For this review, use the dimensioned drawing (mm, ordinates from the lowest corner) and the shaded views. A direction names the side the tool comes from. Coordinates: 2 decimals unless noted, no trailing zeros. Order: outer loops, then holes, each group sorted by start corner. A loop starts at its lowest first (then second) coordinate and runs counter-clockwise, first axis right, second up. Notation, with made-up numbers: M 41.25,22.25 L 83.25,22.25 A3 ccw 83.25,27.25 Z; hole C 65,11 d1. An arc over 180 degrees is marked long. Answer in a Markdown table with one row per item.
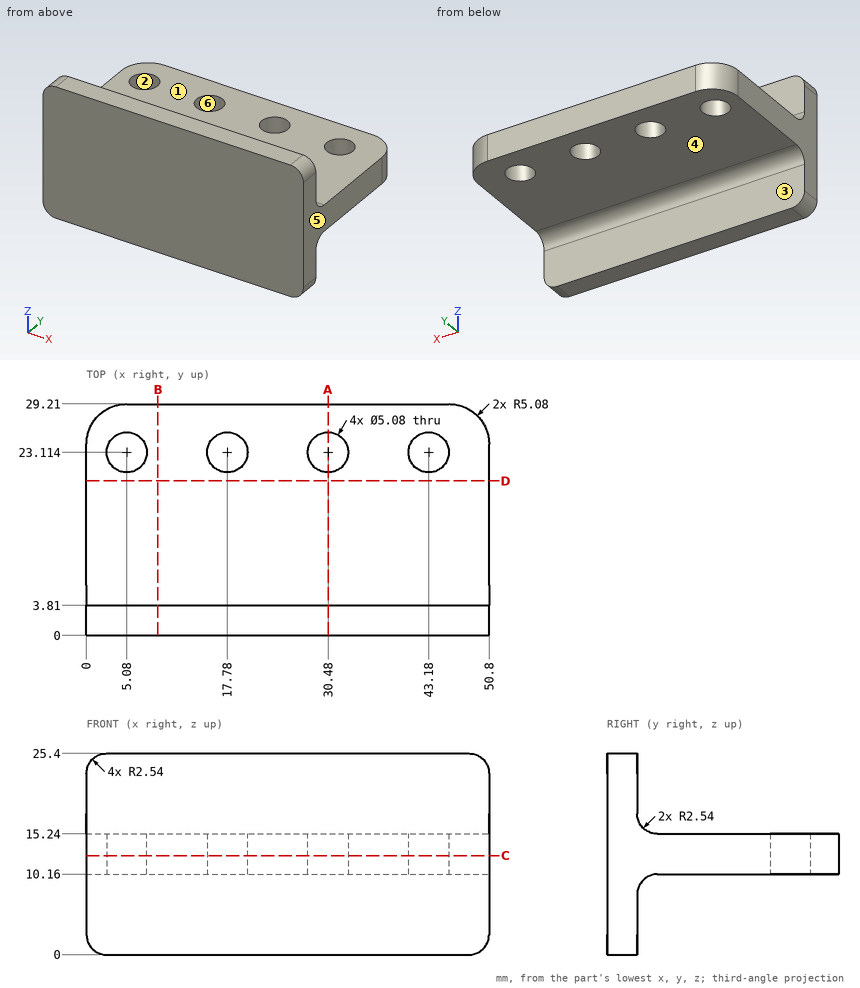
(1) Draft analysis for pull direction X (two halves, no side actions). For the marked faces 4, 5 and 6, state which applies: pulls with the +X half, pulls with the -X half, needs draft (parallel to the pull), parting line crosses it, or undercut.
Return value:
| item | result |
|---|---|
| face 4 | needs draft |
| face 5 | pulls with the +X half |
| face 6 | undercut |
(2) Insertion check: pin 1 Ø3 at (x, z) = (21.5, 20.5) entering from +Y; pin 2 Ø7 at (x, y) = (14, 13) entering from -Z; pin 3 Ø8 at (x, y) = (17.78, 23.114) entering from +Z. Each pin has a flat end and moves straight along its axis. Give the tip position at first contact, or say it passes through.
Return value:
| item | result |
|---|---|
| pin 1 | stops at y = 3.81 |
| pin 2 | stops at z = 10.16 |
| pin 3 | stops at z = 15.24 |
(3) Add section D-D, the plane y = 19.5. Give the boundary of the cut face in (x, z).
Return value:
| item | result |
|---|---|
| outline | M 0,10.16 L 50.8,10.16 L 50.8,15.24 L 0,15.24 Z |
(4) For the marked faces 1, 2 and 3, list the 3-axis set-ups (+Z, -Z, +X, -X, +Y, -Y) from which the entire face can be reached by the end or side of a thin tool; tool diameter is ignored.
Return value:
| item | result |
|---|---|
| face 1 | +Z, +X, -X, +Y |
| face 2 | +Z, -Z |
| face 3 | -Z, +X, -X, +Y |
(5) Add section A-A, the plane x = 30.48. Give the boundary of the cut face in (y, z).
Return value:
| item | result |
|---|---|
| outline | M 0,0 L 3.81,0 L 3.81,7.62 A2.54 cw 6.35,10.16 L 20.57,10.16 L 20.57,15.24 L 6.35,15.24 A2.54 cw 3.81,17.78 L 3.81,25.4 L 0,25.4 Z; M 25.65,10.16 L 29.21,10.16 L 29.21,15.24 L 25.65,15.24 Z |
(6) Add section C-C, the plane z = 12.5. Give the boundary of the cut face in (x, y), and give its area (3 significant figures).
Return value:
| item | result |
|---|---|
| outline | M 0,0 L 50.8,0 L 50.8,24.13 A5.08 ccw 45.72,29.21 L 5.08,29.21 A5.08 ccw 0,24.13 Z; hole C 5.08,23.11 d5.08; hole C 17.78,23.11 d5.08; hole C 30.48,23.11 d5.08; hole C 43.18,23.11 d5.08 |
| area | 1,390 mm2 |
(7) For line 1 along Y through (x, z) = (5.08, 13.65); line 2 along Y through (x, z) = (37, 5.5); line 3 along Z through (x, y) = (22.5, 18.75), list the stretches that pass through material, from the lowest coordinate up. Write a range as from..to.
Return value:
| item | result |
|---|---|
| line 1 | y = 0..20.57, 25.65..29.21 |
| line 2 | y = 0..3.81 |
| line 3 | z = 10.16..15.24 |
(8) Add section B-B, the plane x = 9. Give the boundary of the cut face in (y, z), and give its area (3 significant figures).
Return value:
| item | result |
|---|---|
| outline | M 0,0 L 3.81,0 L 3.81,7.62 A2.54 cw 6.35,10.16 L 29.21,10.16 L 29.21,15.24 L 6.35,15.24 A2.54 cw 3.81,17.78 L 3.81,25.4 L 0,25.4 Z |
| area | 229 mm2 |
